Part print with two shaded views. Sizes in mm from the minimum x, y, z corner. Give positions to 0.01 mm unless a question says otherwise; leave off trailing zeros. Order: outer loops, then holes, each group sorted by start corner. A loop starts at its lowest first (then second) coordinate and runs counter-clockwise, first axis right, second up. Notation, with made-up numbers: M 60.5,20.25 L 105.5,20.25 A25 cw 105.5,54.25 Z; hole C -31.75,-27 d1. An arc over 180 degrees is marked long. Return JSON: item names as keys, results as strings.
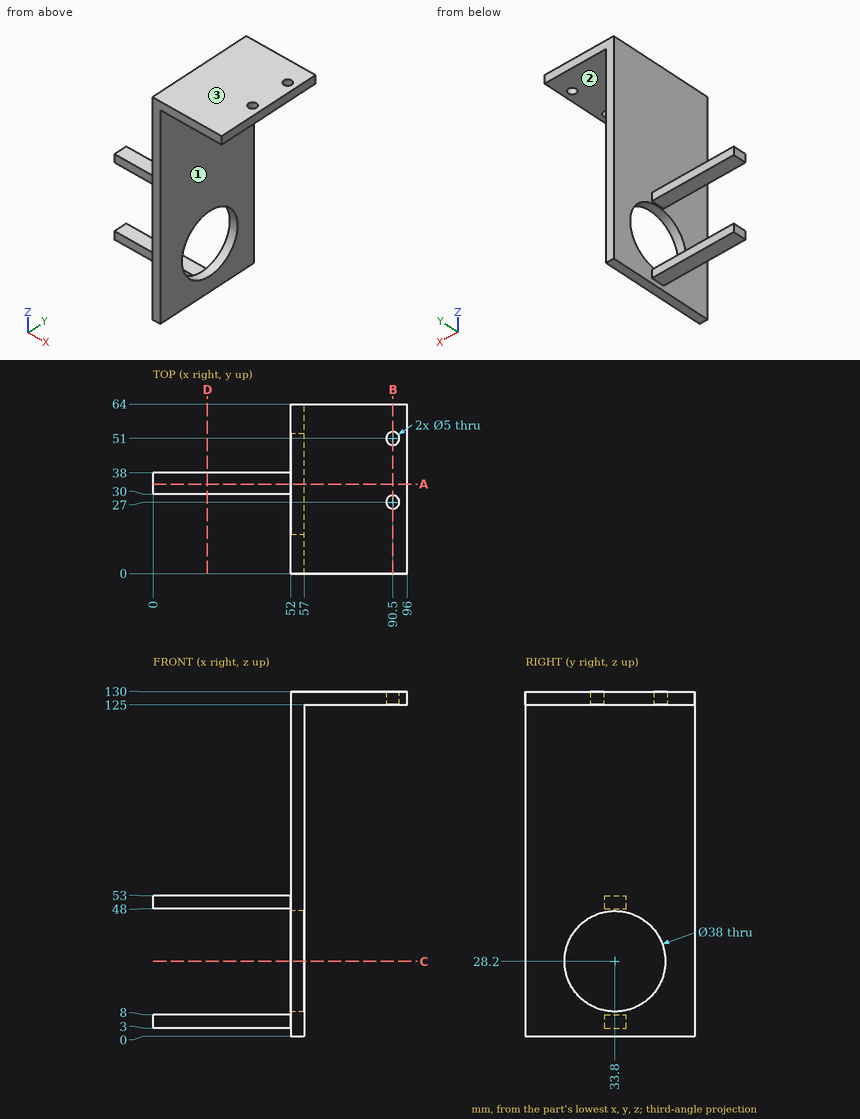
Q1. Pin check, flat tips, straight feed: pin 1 (6.5 mm diameter, centred on x = 13, y = 32.5, fed in from +Z); pin 2 (1.5 mm diameter, centred on y = 39.5, z = 50, fed in from +X); pin 3 (3 mm diameter, centred on x = 51, y = 14, fed in from -Z); pin 4 (4.5 mm diameter, centred on x = 90.5, y = 51, fed in from -Z). Stop position of each tip, or through.
Established:
{"pin 1": "stops at z = 53", "pin 2": "stops at x = 57", "pin 3": "stops at z = 0", "pin 4": "passes through"}
Q2. Band-saw the part on A-A (y = 33.8). Give the cut face in (x, z).
Established:
{"outline": "M 0,3 L 52,3 L 52,0 L 57,0 L 57,9.2 L 52,9.2 L 52,8 L 0,8 Z; M 0,48 L 52,48 L 52,47.2 L 57,47.2 L 57,125 L 96,125 L 96,130 L 52,130 L 52,53 L 0,53 Z"}
Q3. Probe line 1 along Y through (x, z) = (90.5, 128.8); line 2 along Z through (x, y) = (13, 34); line 3 along Y through (x, z) = (55, 28). List the from-to ranges inside material, lowest first.
Established:
{"line 1": "y = 0 to 24.5, 29.5 to 48.5, 53.5 to 64", "line 2": "z = 3 to 8, 48 to 53", "line 3": "y = 0 to 14.8, 52.8 to 64"}
Q4. Band-saw the part on D-D (x = 20.5). Give the cut face in (y, z).
Established:
{"outline": "M 30,3 L 38,3 L 38,8 L 30,8 Z; M 30,48 L 38,48 L 38,53 L 30,53 Z"}
Q5. Band-saw the part on C-C (z = 28.2). Give the cut face in (x, y), then the cut area to 3 significant figures.
Established:
{"outline": "M 52,0 L 57,0 L 57,14.8 L 52,14.8 Z; M 52,52.8 L 57,52.8 L 57,64 L 52,64 Z", "area": "130 mm²"}
Q6. Two-plate mould, pull along Z, no slides. Class the marked faces 1, 2 and 3: +Z half, -Z half, draft (parallel to the pull), parting line (faces both ways), or undercut.
Established:
{"face 1": "draft", "face 2": "-Z half", "face 3": "+Z half"}
Q7. Band-saw the part on B-B (x = 90.5). Give the cut face in (y, z), then the cut area to 3 significant figures.
Established:
{"outline": "M 0,125 L 24.5,125 L 24.5,130 L 0,130 Z; M 29.5,125 L 48.5,125 L 48.5,130 L 29.5,130 Z; M 53.5,125 L 64,125 L 64,130 L 53.5,130 Z", "area": "270 mm²"}
